from build123d import *

# Parameters (mm, degrees)
F1_DEPTH = 25


with BuildPart() as f1:
    # F0 (on Front) → F1 (new body)
    with BuildSketch(Plane.XZ):
        with BuildLine():
            Line((-64.745709, 61.124308), (-64.745709, -23.875692))
            Line((-64.745709, -23.875692), (-52.245709, -23.875692))
            Line((-52.245709, -23.875692), (-52.245709, -20.875692))
            ThreePointArc((-52.245709, -20.875692), (-52.831495, -19.461478), (-54.245709, -18.875692))
            Line((-54.245709, -18.875692), (-59.745709, -18.875692))
            ThreePointArc((-59.745709, -18.875692), (-61.159922, -18.289905), (-61.745709, -16.875692))
            Line((-61.745709, -16.875692), (-61.745709, 3.124308))
            ThreePointArc((-61.745709, 3.124308), (-61.159922, 4.538522), (-59.745709, 5.124308))
            Line((-59.745709, 5.124308), (-59.745709, 42.445086))
            ThreePointArc((-59.745709, 42.445086), (-58.9421, 44.047786), (-57.177062, 44.362543))
            Line((-57.177062, 44.362543), (97.500285, -1.509033))
            ThreePointArc((97.500285, -1.509033), (98.70368, -2.047171), (99.72461, -2.881111))
            Line((99.72461, -2.881111), (127.108349, -32.060611))
            ThreePointArc((127.108349, -32.060611), (128.129279, -32.89455), (129.332675, -33.432689))
            Line((129.332675, -33.432689), (160.254291, -42.602896))
            ThreePointArc((160.254291, -42.602896), (159.406122, -39.3547), (156.694794, -37.375087))
            Line((156.694794, -37.375087), (131.508298, -29.905705))
            ThreePointArc((131.508298, -29.905705), (130.304903, -29.367566), (129.283973, -28.533627))
            Line((129.283973, -28.533627), (101.900234, 0.645873))
            ThreePointArc((101.900234, 0.645873), (100.879304, 1.479812), (99.675908, 2.017951))
            Line((99.675908, 2.017951), (-53.588942, 47.470632))
            ThreePointArc((-53.588942, 47.470632), (-58.759208, 51.075958), (-60.745709, 57.057917))
            Line((-60.745709, 57.057917), (-60.745709, 57.124308))
            ThreePointArc((-60.745709, 57.124308), (-61.917281, 59.952736), (-64.745709, 61.124308))
        make_face()
    extrude(amount=F1_DEPTH)


solid = f1.part
Verification items for the finished model (mm, model axes). A direction names the side the tool comes from. Give positions to 0.01 mm unless a question says otherwise; leave off trailing zeros. Order: outer loops, then holes, each group sorted by start corner. A loop starts at its lowest first (then second) coordinate and runs counter-clockwise, first axis right, second up. Notation, with made-up numbers: M 13,55.5 L 20,55.5 A9 ccw 20,67.5 Z; hole C 39,-22.5 d9. An arc over 180 degrees is marked long. Answer as a JSON object with one key per item and string values. Group by question number.
1) Access from +Z, -Z, +X, -X, +Y, -Y to the whole of each face (thin tool, end or side, straight path). Record for faces 5 (the face through (-59, -12, -23.876)), 6 (the face through (22.2, -25, 21)), 7 (the face through (-57, -12, -18.876)).
2) Cross-section at D-D (z = 38). Enter the section's corners in (x, y).
3) Depth check by flat-ended pin: pin 1 Ø2 at (y, z) = (-7, -31.5) entering from -X; pin 2 Ø3 at (x, y) = (-15.5, -9) entering from -Z; pin 3 Ø1.5 at (y, z) = (-15, -24.5) entering from +X. Enter the tip coordinate at first touch or a pass-through.
4) Cross-section at C-C (x = -1). Enter the section's corners in (y, z).
5) Mould release check, pull along Z, two halves, no side actions. Record for faces 1 (the face through (-59.746, -12, 24)), 2 (the face through (113.225, -12.325, -17.267)), 3 (the face through (-61.746, -12, -7)), 4 (the face through (24.116, -12.325, 24.426)): released by +Z, released by -Z, zero draft, split by the parting line, or undercut.
6) Cross-section at A-A (z = -6.5). Enter the section's corners in (x, y).
7) Scan lines: line 1 along X through (y, z) = (-1, -18.5); line 2 along X through (y, z) = (-23.5, -22); line 3 along Z through (x, y) = (90.5, -14.75). Record each from-to range of solid material in increasing order. Write a range as [from, to].
8) Cross-section at B-B (y = -17.75). Enter the section's corners in (x, z), then the cut area to 3 significant figures.
Result sheet:
{
 "1": {"face 5": "-Z, -X, +Y, -Y", "face 6": "+Z, -Z, +X, -X, -Y", "face 7": "+Y, -Y"},
 "2": {"outline": "M -64.75,-25 L -59.75,-25 L -59.75,0 L -64.75,0 Z; M -35.72,-25 L -21.65,-25 L -21.65,0 L -35.72,0 Z"},
 "3": {"pin 1": "stops at x = 125.64", "pin 2": "stops at z = 31.56", "pin 3": "stops at x = 126.2"},
 "4": {"outline": "M -25,27.7 L 0,27.7 L 0,31.87 L -25,31.87 Z"},
 "5": {"face 1": "undercut", "face 2": "released by -Z", "face 3": "undercut", "face 4": "released by +Z"},
 "6": {"outline": "M -64.75,-25 L -61.75,-25 L -61.75,0 L -64.75,0 Z; M 103.12,-25 L 108.61,-25 L 108.61,0 L 103.12,0 Z"},
 "7": {"line 1": "x = [-64.75, -60.91], [114.38, 119.87]", "line 2": "x = [-64.75, -52.25], [117.67, 123.15]", "line 3": "z = [0.57, 4.74]"},
 "8": {"outline": "M -64.75,-23.88 L -52.25,-23.88 L -52.25,-20.88 A2 ccw -54.25,-18.88 L -59.75,-18.88 A2 cw -61.75,-16.88 L -61.75,3.12 A2 cw -59.75,5.12 L -59.75,42.45 A2 cw -57.18,44.36 L 97.5,-1.51 A5 cw 99.72,-2.88 L 127.11,-32.06 A5 ccw 129.33,-33.43 L 160.25,-42.6 A5 ccw 156.69,-37.38 L 131.51,-29.91 A5 cw 129.28,-28.53 L 101.9,0.65 A5 ccw 99.68,2.02 L -53.59,47.47 A10 cw -60.75,57.06 L -60.75,57.12 A4 ccw -64.75,61.12 Z", "area": "1,380 mm2"}
}
